For this review, take the finished solid that the model builds, in its own axes (mm). A direction names the side the tool comes from. Give positions to 0.01 mm unless a question says otherwise; leave off trailing zeros. Order: outer loops, then holes, each group sorted by start corner. A loop starts at its lowest first (then second) coordinate and runs counter-clockwise, first axis right, second up.
Item 1: For P1, Ø5, axis at x = 4.5, z = 54, coming from the +Y side; P2, Ø5, axis at x = 9, y = -8.5, coming from the -Z side, all flat-tipped, find the tip position at first contact; note any pin that passes through.
Item 2: The part is to be moulded in two halves that separate along X. For faces 4 (the flat face through (10, 0, 1)), 5 (the cylindrical face through (6.187, -30.07, -49.636)), 6 (the cylindrical face through (4.93, 26.014, 23.28)), say which applies: released by +X, released by -X, zero draft, split by the parting line, or undercut.
Item 3: Machinability: for faces 1 (the flat face through (5, 0, 45)), 2 (the flat face through (5, -25, -56)), 3 (the flat face through (0, 0, 1)), which of the approach directions +Z, -Z, +X, -X, +Y, -Y give a long, thin tool a straight path to every point of the face, cutting with its end or side? Answer none if there is none.
Item 4: Consider section A-A (z = 52.5). Give the boundary of the cut face in (x, y), plus the area to 3 significant figures.
Item 5: For probe 1 along Y at (x, z) = (5, -22.5); probe 2 along Z at (x, y) = (7.25, 22.5); probe 3 along X at (y, z) = (-27.25, 52.5), list the stretches that pass through material, from the lowest coordinate up.
Item 6: Consider section C-C (z = -22.5). Give the boundary of the cut face in (x, y), plus the area to 3 significant figures.
Item 7: Consider section B-B (y = -22.5). Give the boundary of the cut face in (x, z), plus the area to 3 significant figures.
Item 8: Consider section D-D (x = 3.5). Give the number of separate pieces and of enclosed holes in the cut face, plus the area to 3 significant figures.
Autodesk Inventor part; units mm, degrees
ref_plane "YZ Plane" through (0, 0, 0) normal (1, 0, 0) x (0, 1, 0)
ref_plane "XZ Plane" through (0, 0, 0) normal (0, 1, 0) x (-1, 0, 0)
ref_plane "XY Plane" through (0, 0, 0) normal (0, 0, 1) x (1, 0, 0)
sketch "Sketch1" plane through (0, 0, 0) normal (1, 0, 0) x (0, 1, 0)
  line L0 (-35, 60) -> (35, 60)
  line L1 (35, 60) -> (35, -60)
  line L2 (35, -60) -> (-35, -60)
  line L3 (-35, -60) -> (-35, 60)
  line L4 (-35, 60) -> (35, -60) construction
  line L5 (35, 60) -> (-35, -60) construction
  line L6 (0, 60) -> (0, -60) construction
  line L7 (20, 60) -> (35, -15)
  line L8 (0, 22.5) -> (0, -22.5)
  line L9 (-35, 0) -> (35, 0) construction
  circle A0 centre (0, 22.5) radius 18 construction
  circle A1 centre (0, -22.5) radius 26 construction
  line L10 (-35, 51) -> (35, 51)
  circle A2 centre (0, 22.5) radius 6
  circle A3 centre (0, -22.5) radius 6
  point P0 (0, 0)
  point P1 (21.8, 51)
  dimension "d0" = 35
  dimension "d1" = 120
  dimension "d2" = 45
  dimension "d3" = 52
  dimension "d4" = 36
  dimension "d5" = 75
  dimension "d6" = 15
  dimension "d7" = 9
  dimension "d8" = 12
  dimension "d9" = 12
extrude "Extrusion1" add sketch "Sketch1" along normal blind 10
sketch "Sketch2" plane through (0, 35, -15) normal (0, 1, 0) x (1, 0, 0)
  line L0 (0, 45) -> (0, -75) construction
  line L1 (10, 45) -> (10, -75)
  line L2 (0, 45) -> (10, 45)
  line L3 (0, 0) -> (0, -66)
  line L4 (0, -66) -> (10, -66) construction
  line L5 (10, 0) -> (10, -66)
  line L6 (0, 0) -> (10, 0)
  line L7 (0, 45) -> (10, 45)
  line L8 (0, 45) -> (10, 45)
  line L9 (10, 45) -> (10, 30)
  line L10 (10, 30) -> (0, 30)
  line L11 (0, 30) -> (0, 45)
  line L12 (0, -75) -> (10, -75)
  line L13 (0, 45) -> (0, -75)
  line L14 (0, -75) -> (10, -75)
  line L15 (10, -75) -> (10, -60)
  line L16 (10, -60) -> (0, -60)
  line L17 (0, -60) -> (0, -75)
  point P0 (0, -15)
  point P1 (0, 30)
  point P2 (0, -60)
  dimension "d36" = 15
  dimension "d37" = 15
extrude "Extrusion2" cut sketch "Sketch2" against normal blind 60 contours L1 L10 L11 L2 | L1 L12 L13 L3 L16
sketch "Sketch3" plane through (10, 0, 0) normal (1, 0, 0) x (0, 0, -1)
  line L0 (45, 35) -> (-45, 35)
  line L1 (-60, -35) -> (60, -35)
  line L2 (60, -35) -> (60, -25)
  circle A0 centre (-22.5, 0) radius 6
  circle A1 centre (22.5, 0) radius 6
  line L3 (-22.5, 22.5) -> (-22.5, -22.5)
  line L4 (-22.5, 0) -> (22.5, 0) construction
  line L5 (22.5, 22.5) -> (22.5, -22.5)
  line L6 (-60, -25) -> (-60, -35)
  line L7 (45, -25) -> (45, 35)
  line L8 (-45, 35) -> (-45, -25)
  line L9 (-45, -25) -> (-60, -25)
  line L10 (60, -25) -> (45, -25)
  point P0 (0, 0)
  dimension "d16" = 45
hole "Hole1" at (10, 22.5, 22.5) at (10, -22.5, 22.5) at (10, 22.5, -22.5) at (10, -22.5, -22.5) direction (-1, 0, 0) diameter 7.2 end through all
sketch "Sketch4" plane through (0, -25, -15) normal (0, 1, 0) x (1, 0, 0)
  line L0 (0, 30) -> (0, 45)
  line L1 (10, -60) -> (10, -75)
  line L2 (10, 45) -> (10, 30)
  line L3 (0, 45) -> (10, 45)
  line L4 (0, 30) -> (0, 45)
  line L5 (10, 30) -> (0, 30)
  line L6 (5, -75) -> (5, 45)
  line L7 (10, 45) -> (10, 30)
  line L8 (0, 45) -> (10, 45)
  line L9 (10, 30) -> (0, 30)
  line L10 (0, -75) -> (0, -60)
  line L11 (10, -75) -> (0, -75)
  line L12 (0, -60) -> (10, -60)
  point P0 (0, -15)
  point P1 (5, -67.5)
  point P2 (5, 37.5)
  dimension "d24" = 7.5
  dimension "d38" = 7.5
hole "Hole2" at (5, -25, 52.5) at (5, -25, -52.5) direction (0, -1, 0) diameter 6.2 end through all
chamfer "Chamfer1" distance 10 angle 45 2 edges at (5, 35, -45) (5, 35, 45)
properties part number "22_Hop_so_ngang" material "Stainless Steel, Austenitic"
Resolved:
1. P1: stops at y = -25
1. P2: stops at z = -45
2. face 4: released by +X
2. face 5: undercut
2. face 6: zero draft
3. face 1: +Z, +X, -X, +Y
3. face 2: -Z, +X, -X, +Y
3. face 3: +Z, -Z, -X, +Y, -Y
4. outline: (0, -35) - (1.9, -35) - (1.9, -25) - (0, -25) - close; (8.1, -35) - (10, -35) - (10, -25) - (8.1, -25) - close
4. area: 38.0 mm2
5. probe 1: y = -35 to -26.1, -18.9 to -6, 6 to 18.9, 26.1 to 35
5. probe 2: z = -45 to -26.1, -18.9 to 18.9, 26.1 to 45
5. probe 3: x = 0 to 1.9, 8.1 to 10
6. outline: (0, -35) - (10, -35) - (10, -26.1) - (0, -26.1) - close; (0, -18.9) - (10, -18.9) - (10, -6) - (0, -6) - close; (0, 6) - (10, 6) - (10, 18.9) - (0, 18.9) - close; (0, 26.1) - (10, 26.1) - (10, 35) - (0, 35) - close
6. area: 436 mm2
7. outline: (0, -45) - (10, -45) - (10, -26.1) - (0, -26.1) - close; (0, -18.9) - (10, -18.9) - (10, 18.9) - (0, 18.9) - close; (0, 26.1) - (10, 26.1) - (10, 45) - (0, 45) - close
7. area: 756 mm2
8. separate pieces: 3
8. enclosed holes: 6
8. area: 6,000 mm2
